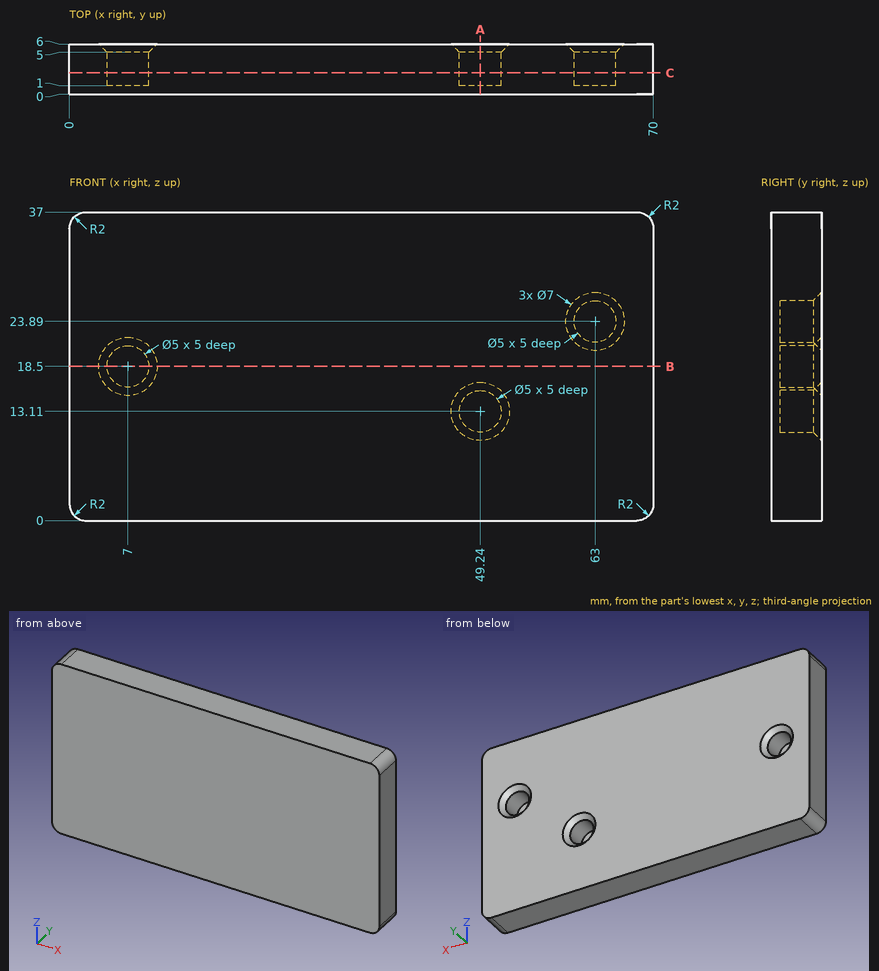
The figure shows three views and two pictorial views of one solid part (mm, origin at its lowest corner). Answer the questions. Coordinates: 2 decimals unless noted, no trailing zeros. Order: outer loops, then holes, each group sorted by start corner. A loop starts at its lowest first (then second) coordinate and runs counter-clockwise, first axis right, second up.
Q1. Consider line 1 (X direction, y = 2.75, z = 13.11); line 2 (X direction, y = 3.55, z = 18.5); line 3 (X direction, y = 5.7, z = 16). Determine where each line is inside the solid, lowest interval first.
Q2. A cutting plane is placed at A-A, the plane x = 49.24. Write down the section's boundary in (y, z), and give its area (3 significant figures).
Q3. A cutting plane is placed at C-C, the plane y = 2.55. Write down the section's boundary in (x, z), and give its area (3 significant figures).
Q4. A cutting plane is placed at B-B, the plane z = 18.5. Write down the section's boundary in (x, y).
Q5. Given P1, Ø6, axis at x = 63, z = 23.89, coming from the +Y side; P2, Ø4, axis at x = 63.5, z = 24.5, coming from the +Y side; P3, Ø1.5, axis at x = 48.5, z = 12.5, coming from the +Y side, each flat-ended and moving along its own axis, determine where each tip first touches the part or whether it passes through.
Answers follow:
1. line 1: x = 0 to 46.74, 51.74 to 70
1. line 2: x = 0 to 4.5, 9.5 to 70
1. line 3: x = 0 to 5, 9 to 47.87, 50.61 to 70
2. outline: (0, 0) - (6, 0) - (6, 9.61) - (5, 10.61) - (1, 10.61) - (1, 15.61) - (5, 15.61) - (6, 16.61) - (6, 37) - (0, 37) - close
2. area: 196 mm2
3. outline: (0, 2) arc R2 ccw to (2, 0) - (68, 0) arc R2 ccw to (70, 2) - (70, 35) arc R2 ccw to (68, 37) - (2, 37) arc R2 ccw to (0, 35) - close; hole circle Ø5 at (7, 18.5); hole circle Ø5 at (49.24, 13.11); hole circle Ø5 at (63, 23.89)
3. area: 2,530 mm2
4. outline: (0, 0) - (70, 0) - (70, 6) - (10.5, 6) - (9.5, 5) - (9.5, 1) - (4.5, 1) - (4.5, 5) - (3.5, 6) - (0, 6) - close
5. P1: stops at y = 5.5
5. P2: stops at y = 5.29
5. P3: stops at y = 1
